The model under review builds one solid part; all positions refer to its coordinate system, in mm. Face numbers are marked on the shaded views. A direction names the side the tool comes from. Give positions to 0.01 mm unless a question says otherwise; leave off trailing zeros. Order: outer loops, then holes, each group sorted by start corner. A loop starts at its lowest first (then second) coordinate and runs counter-clockwise, first axis right, second up. Notation, with made-up numbers: (38.5, 78) - (82.5, 78) arc R18 cw to (82.5, 92) - close; hole circle Ø1 at (-16.5, 87.25). An arc over 180 degrees is marked (long way). Use CSV: the item, a comma, the result in double quotes. Start each with the question number.
1. Take a section at B-B, the plane x = 0. State the section outline as (y, z) points (3 decimals).
2. Take a section at A-A, the plane z = 0. State the section outline as (x, y) points (3 decimals).
3. Take a section at D-D, the plane z = -14.5. State the section outline as (x, y) points, then the cut area to 3 significant figures.
4. Machinability: for the marked faces 4 and 5, which of the approach directions +Z, -Z, +X, -X, +Y, -Y give a long, thin tool a straight path to every point of the face, cutting with its end or side? Answer none if there is none.
5. For pin 1 (3 mm diameter, centred on x = 16, y = 4.5, fed in from -Z); pin 2 (1 mm diameter, centred on x = 10, y = 3.5, fed in from -Z); pin 3 (3 mm diameter, centred on x = -19.5, y = 4, fed in from +Z); pin 4 (5 mm diameter, centred on x = 0, z = 0, fed in from +Y), all flat-tipped, find the tip position at first contact; note any pin that passes through.
6. Draft analysis for pull direction Z (two halves, no side actions). For the marked faces 1, 2 and 3, state which applies: released by +Z, released by -Z, zero draft, split by the parting line, or undercut.
7. Take a section at C-C, the plane y = 1.25. State the section outline as (x, z) points (3 decimals), then the cut area to 3 significant figures.
8. To check wall thickness, follow line 1 (Z direction, x = -14, y = 3.75); line 2 (Z direction, x = 20, y = 5.75); line 3 (X direction, y = 3, z = 0) (3 decimals). State the ranges of each line that lie inside material, in increasing order. Write a range as [from, to].
```python
from build123d import *

# Parameters (mm, degrees)
SKETCH1_R           = 30
BOSS_EXTRUDE1_DEPTH = 6.35
SKETCH2_R           = 3.175
CUT_EXTRUDE1_DEPTH  = 43.898980174
CUT_EXTRUDE2_DEPTH  = 43.898980174


with BuildPart() as part:
    # Sketch1 → Boss-Extrude1 (new body)
    with BuildSketch(Plane(origin=(0, 0, 0), x_dir=(1, 0, 0), z_dir=(0, 1, 0))):
        with Locations(Location((0, 0, 0), (0, 0, 270))):
            Circle(SKETCH1_R)
    extrude(amount=BOSS_EXTRUDE1_DEPTH)

    # Sketch2 → Cut-Extrude1 (cut, through all)
    with BuildSketch(Plane(origin=(0, 6.35, 0), x_dir=(1, 0, 0), z_dir=(0, 1, 0))):
        with Locations(Location((0, 0, 0), (0, 0, 270))):
            Circle(SKETCH2_R)
    extrude(amount=-CUT_EXTRUDE1_DEPTH, mode=Mode.SUBTRACT)

    # Sketch3 → Cut-Extrude2 (cut, through all)
    with BuildSketch(Plane(origin=(0, 6.35, 0), x_dir=(1, 0, 0), z_dir=(0, 1, 0))):
        with BuildLine():
            Line((8.89, -2.54), (25.4, -2.54))
            ThreePointArc((25.4, -2.54), (18.076447857, -18.076447857), (2.54, -25.4))
            Line((2.54, -25.4), (2.54, -8.89))
            ThreePointArc((2.54, -8.89), (6.53772514, -6.53772514), (8.89, -2.54))
        make_face()
        with BuildLine():
            Line((-2.54, -8.89), (-2.54, -25.4))
            ThreePointArc((-2.54, -25.4), (-17.845937126, -17.845937126), (-25.4, -2.54))
            Line((-25.4, -2.54), (-8.89, -2.54))
            ThreePointArc((-8.89, -2.54), (-6.53772514, -6.53772514), (-2.54, -8.89))
        make_face()
        with BuildLine():
            Line((-8.89, 2.54), (-25.4, 2.54))
            ThreePointArc((-25.4, 2.54), (-17.794170178, 17.794170178), (-2.54, 25.4))
            Line((-2.54, 25.4), (-2.54, 8.89))
            ThreePointArc((-2.54, 8.89), (-6.53772514, 6.53772514), (-8.89, 2.54))
        make_face()
        with BuildLine():
            Line((2.54, 8.89), (2.54, 25.4))
            ThreePointArc((2.54, 25.4), (17.845937126, 17.845937126), (25.4, 2.54))
            Line((25.4, 2.54), (8.89, 2.54))
            ThreePointArc((8.89, 2.54), (6.53772514, 6.53772514), (2.54, 8.89))
        make_face()
    extrude(amount=-CUT_EXTRUDE2_DEPTH, mode=Mode.SUBTRACT)


solid = part.part
```
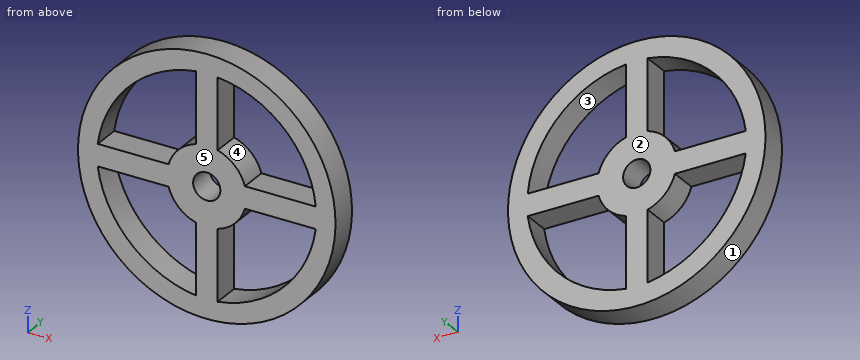
Determined:
1,outline,"(0, -30) - (6.35, -30) - (6.35, -3.175) - (0, -3.175) - close; (0, 3.175) - (6.35, 3.175) - (6.35, 30) - (0, 30) - close"
2,outline,"(-30, 0) - (-3.175, 0) - (-3.175, 6.35) - (-30, 6.35) - close; (3.175, 0) - (30, 0) - (30, 6.35) - (3.175, 6.35) - close"
3,outline,"(-26.26, 0) - (-20.6, 0) - (-20.6, 6.35) - (-26.26, 6.35) - close; (-2.54, 0) - (2.54, 0) - (2.54, 6.35) - (-2.54, 6.35) - close; (20.68, 0) - (26.26, 0) - (26.26, 6.35) - (20.68, 6.35) - close"
3,area,"104 mm²"
4,face 4,"+Y, -Y"
4,face 5,"+Z, -Z, +X, -X, -Y"
5,pin 1,"stops at z = -26.26"
5,pin 2,"stops at z = -28.46"
5,pin 3,"stops at z = 24"
5,pin 4,"passes through"
6,face 1,"split by the parting line"
6,face 2,"zero draft"
6,face 3,"undercut"
7,outline,"circle Ø60 at (0, 0); hole (-25.4, -2.54) arc R26.861 ccw to (-2.54, -25.4) - (-2.54, -8.89) arc R9.246 cw to (-8.89, -2.54) - close; hole (-25.4, 2.54) - (-8.89, 2.54) arc R9.246 cw to (-2.54, 8.89) - (-2.54, 25.4) arc R26.575 ccw to start; hole circle Ø6.35 at (0, 0); hole (2.54, -25.4) arc R26.575 ccw to (25.4, -2.54) - (8.89, -2.54) arc R9.246 cw to (2.54, -8.89) - close; hole (2.54, 8.89) arc R9.246 cw to (8.89, 2.54) - (25.4, 2.54) arc R25.4 ccw to (2.54, 25.4) - close"
7,area,"1,370 mm²"
8,line 1,"z = [-26.53, -20.95], [-2.54, 2.54], [21.03, 26.53]"
8,line 2,"z = [-22.36, -15.41], [-2.54, 2.54], [15.92, 22.36]"
8,line 3,"x = [-30, -3.175], [3.175, 30]"
